Geometry: final body of the model. Coordinates: model frame, mm. A direction names the side the tool comes from. Coordinates: 2 decimals unless noted, no trailing zeros. Loops run counter-clockwise (first coordinate to the right, second up) from the corner with the lowest first, then second, coordinate; pieces in that order, holes last. Notation, with made-up numbers: (41.25, 64) - (93.25, 64) arc R22 ccw to (93.25, 80) - close; hole circle Ø11 at (70, 34). An arc over 180 degrees is marked (long way). Answer in a Markdown table with one row per item.
from build123d import *

# Parameters (mm, degrees)
SKETCH1_W           = 88.9
SKETCH1_H           = 78.74
SKETCH1_R           = 1.5
BOSS_EXTRUDE1_DEPTH = 1.5
SKETCH2_W           = 58.4
SKETCH2_H           = 17.9
BOSS_EXTRUDE2_DEPTH = 14.72
SKETCH3_W           = 30.2
SKETCH3_H           = 8.2
BOSS_EXTRUDE3_DEPTH = 9.65
SKETCH4_R           = 6.625
BOSS_EXTRUDE6_DEPTH = 25.4


with BuildPart() as part:
    # Sketch1 → Boss-Extrude1 (new body)
    with BuildSketch(Plane(origin=(0, 0, 0), x_dir=(1, 0, 0), z_dir=(0, 1, 0))):
        Rectangle(SKETCH1_W, SKETCH1_H)
        with Locations((-41.91, 36.83)):
            Circle(SKETCH1_R, mode=Mode.SUBTRACT)
        with Locations((41.91, 36.83)):
            Circle(SKETCH1_R, mode=Mode.SUBTRACT)
        with Locations((41.91, -36.83)):
            Circle(SKETCH1_R, mode=Mode.SUBTRACT)
        with Locations((-41.91, -36.83)):
            Circle(SKETCH1_R, mode=Mode.SUBTRACT)
    extrude(amount=BOSS_EXTRUDE1_DEPTH)

    # Sketch2 → Boss-Extrude2 (add)
    with BuildSketch(Plane(origin=(0, 1.5, 0), x_dir=(1, 0, 0), z_dir=(0, 1, 0))):
        with Locations((0, 28.09)):
            Rectangle(SKETCH2_W, SKETCH2_H)
    extrude(amount=BOSS_EXTRUDE2_DEPTH)

    # Sketch3 → Boss-Extrude3 (add)
    with BuildSketch(Plane(origin=(0, 1.5, 0), x_dir=(1, 0, 0), z_dir=(0, 1, 0))):
        with Locations((23.69, -35.27)):
            Rectangle(SKETCH3_W, SKETCH3_H)
    extrude(amount=BOSS_EXTRUDE3_DEPTH)

    # Sketch4 → Boss-Extrude6 (add)
    with BuildSketch(Plane(origin=(0, 1.5, 0), x_dir=(1, 0, 0), z_dir=(0, 1, 0))):
        with Locations((-1.125, 10.405)):
            Circle(SKETCH4_R)
        with Locations((-1.125, -2.945)):
            Circle(SKETCH4_R)
    extrude(amount=BOSS_EXTRUDE6_DEPTH)


solid = part.part
(1) Pull-direction query (Z, two-part tool) for faces 4 (the face through (9, 4, 39.37)), 5 (the face through (-2.561, 14.022, 9.412)), 6 (the face through (0, 16.22, -28)); classes: pulls with the +Z half, pulls with the -Z half, needs draft (parallel to the pull), parting line crosses it, or undercut.
Verdict:
| item | result |
|---|---|
| face 4 | pulls with the +Z half |
| face 5 | undercut |
| face 6 | needs draft |
(2) Cut plane C-C on x = 26.5. Output: boundary loops of the cut face in (y, z), then the cut area to 3 significant figures.
Verdict:
| item | result |
|---|---|
| outline | (0, -39.37) - (1.5, -39.37) - (1.5, -37.04) - (16.22, -37.04) - (16.22, -19.14) - (1.5, -19.14) - (1.5, 31.17) - (11.15, 31.17) - (11.15, 39.37) - (0, 39.37) - close |
| area | 461 mm² |
(3) First-contact query: pin 1 Ø9 at (y, z) = (6.5, 34) entering from -X; pin 2 Ø7.5 at (y, z) = (7.5, -25.5) entering from +X; pin 3 Ø2.5 at (x, z) = (24, 37) entering from +Y; pin 4 Ø23.5 at (x, z) = (-13.5, -8.5) entering from +Y. Flat tips, straight axial feed; report the tip coordinate or a pass-through.
Verdict:
| item | result |
|---|---|
| pin 1 | stops at x = 8.59 |
| pin 2 | stops at x = 29.2 |
| pin 3 | stops at y = 11.15 |
| pin 4 | stops at y = 26.9 |
(4) Cut plane A-A on z = 36.83. Output: boundary loops of the cut face in (x, y).
Verdict:
| item | result |
|---|---|
| outline | (-44.45, 0) - (-43.41, 0) - (-43.41, 1.5) - (-44.45, 1.5) - close; (-40.41, 0) - (40.41, 0) - (40.41, 1.5) - (38.79, 1.5) - (38.79, 11.15) - (8.59, 11.15) - (8.59, 1.5) - (-40.41, 1.5) - close; (43.41, 0) - (44.45, 0) - (44.45, 1.5) - (43.41, 1.5) - close |
(5) Cut plane B-B on x = -41.91. Output: boundary loops of the cut face in (y, z).
Verdict:
| item | result |
|---|---|
| outline | (0, -39.37) - (1.5, -39.37) - (1.5, -38.33) - (0, -38.33) - close; (0, -35.33) - (1.5, -35.33) - (1.5, 35.33) - (0, 35.33) - close; (0, 38.33) - (1.5, 38.33) - (1.5, 39.37) - (0, 39.37) - close |
(6) Access query for faces 1 (the face through (-29.2, 9, -28)), 2 (the face through (0, 9, -19.14)), 3 (the face through (29.2, 9, -28)). Directions: +Z, -Z, +X, -X, +Y, -Y. A direction counts if a zero-diameter tool reaches every point of the face in a straight line with its end or side. Return the directions, or none.
Verdict:
| item | result |
|---|---|
| face 1 | +Z, -Z, -X, +Y |
| face 2 | +X, -X, +Y |
| face 3 | -Z, +X, +Y |
(7) Cut plane D-D on y = 12.25. Output: boundary loops of the cut face in (x, z) (3 decimals), then the cut area to 3 significant figures.
Verdict:
| item | result |
|---|---|
| outline | (-29.2, -37.04) - (29.2, -37.04) - (29.2, -19.14) - (-29.2, -19.14) - close; circle Ø13.25 at (-1.125, -10.405); circle Ø13.25 at (-1.125, 2.945) |
| area | 1,320 mm² |
(8) Ray query, probe 1 along Z at (x, y) = (41.91, 0.8); probe 2 along X at (y, z) = (1, -36.83); probe 3 along Z at (x, y) = (23.5, 9.75). Return the intervals inside material, ascending.
Verdict:
| item | result |
|---|---|
| probe 1 | z = -39.37 to -38.33, -35.33 to 35.33, 38.33 to 39.37 |
| probe 2 | x = -44.45 to -43.41, -40.41 to 40.41, 43.41 to 44.45 |
| probe 3 | z = -37.04 to -19.14, 31.17 to 39.37 |
